Design review of the part built by this model. Coordinates are the model's own, in mm. A direction names the side the tool comes from. Coordinates: 2 decimals unless noted, no trailing zeros. Loops run counter-clockwise (first coordinate to the right, second up) from the corner with the lowest first, then second, coordinate; pieces in that order, holes last. Notation, with made-up numbers: (76, 82) -> (133, 82) arc R34 ccw to (133, 120) -> close; hole circle Ø11 at (65, 15.25). An arc over 180 degrees is marked (long way). Use a Markdown table: item, result. Add a question column.
Q1. For faces 1 (the face through (5, 5, 0)), 2 (the face through (5, -0.053, 7)), 3 (the face through (5, 10.947, 7)), 4 (the face through (10.885, 1.234, 7.395)), 5 (the face through (-0.8, 1.17, 7.4)), list the 3-axis set-ups (+Z, -Z, +X, -X, +Y, -Y) from which the entire face can be reached by the end or side of a thin tool; tool diameter is ignored.
Q2. Clearance check with flat-ended pins moving along their axes: pin 1 Ø8 at (y, z) = (-0.5, 8.5) entering from +X; pin 2 Ø1.5 at (x, z) = (0, 11) entering from +Y; pin 3 Ø4.5 at (x, z) = (4, 8.5) entering from +Y; pin 4 Ø6 at (y, z) = (-6, 7) entering from +X. State where each tip first meets the part, or that it passes through.
Q3. Take a section at A-A on z = 11. Write out the cut boundary in (x, y).
Q4. Draft analysis for pull direction X (two halves, no side actions). For faces 6 (the face through (5, 5, -4)), 7 (the face through (11.37, 9.06, 7.4)), 8 (the face through (9.478, 7.42, 7.395)), state which applies: pulls with the +X half, pulls with the -X half, needs draft (parallel to the pull), parting line crosses it, or undercut.
Q5. Take a section at D-D on x = 1. Write out the cut boundary in (y, z).
Q6. Take a section at B-B on x = -2.5. Write out the cut boundary in (y, z), plus the area to 3 significant figures.
Q7. Take a section at C-C on y = -3.5. Write out the cut boundary in (x, z).
Q8. For probe 1 along Y at (x, z) = (4, 5.5); probe 2 along Z at (x, y) = (4.5, -5.5); probe 3 along Y at (x, z) = (0.5, 3.25), list the stretches that pass through material, from the lowest coordinate up.
Solid Edge part; units mm, degrees
sketch "Sketch1" plane through (0, 0, 0) normal (0, 0, 1) x (1, 0, 0)
  arc A0 (-2.9781, 4.4363) -> (3.0001, 10.9473) centre (3.0001, 4.9473) cw
  line L0 (3.0001, 10.9473) -> (7.0001, 10.9473)
  arc A1 (7.0001, 10.9473) -> (12.9783, 4.4363) centre (7.0001, 4.9473) cw
  arc A2 (12.9783, 4.4363) -> (10.4883, 0.9473) centre (7.1717, 5.9473) cw
  arc A3 (10.4883, 0.9473) -> (7.1717, -0.0527) centre (7.1717, 5.9473) cw
  line L1 (7.1717, -0.0527) -> (2.8286, -0.0527)
  arc A4 (2.8286, -0.0527) -> (-0.4881, 0.9473) centre (2.8286, 5.9473) cw
  arc A5 (-0.4881, 0.9473) -> (-2.9781, 4.4363) centre (2.8286, 5.9473) cw
  line L2 (3.0001, 8.4473) -> (7.0001, 8.4473)
  arc A6 (7.0001, 8.4473) -> (10.4991, 4.8617) centre (7.0001, 4.9473) cw
  arc A7 (10.4991, 4.8617) -> (9.1064, 3.0306) centre (7.1717, 5.9473) cw
  arc A8 (9.1064, 3.0306) -> (7.1717, 2.4473) centre (7.1717, 5.9473) cw
  line L3 (7.1717, 2.4473) -> (2.8286, 2.4473)
  arc A9 (2.8286, 2.4473) -> (0.8939, 3.0306) centre (2.8286, 5.9473) cw
  arc A10 (0.8939, 3.0306) -> (-0.4988, 4.8617) centre (2.8286, 5.9473) cw
  arc A11 (-0.4988, 4.8617) -> (3.0001, 8.4473) centre (3.0001, 4.9473) cw
extrude "Protrusion1" add sketch "Sketch1" along normal blind 15
sketch "Sketch2" plane through (5.0001, 5.4473, 0) normal (0, 0, -1) x (1, 0, 0)
  circle A0 centre (-0.0852, 0.1989) radius 15.3143
extrude "ExtrudedProtrusion_2" add sketch "Sketch2" along normal blind 4
Answer list:
| question | item | result |
|---|---|---|
| 1 | face 1 | +Z |
| 1 | face 2 | +Z, +X, -X, -Y |
| 1 | face 3 | +Z, +X, -X, +Y |
| 1 | face 4 | +Z, +X, -Y |
| 1 | face 5 | +Z, -X, -Y |
| 2 | pin 1 | x = 12.65 |
| 2 | pin 2 | y = 10.51 |
| 2 | pin 3 | y = 10.95 |
| 2 | pin 4 | through |
| 3 | outline | (-2.98, 4.44) arc R6 ccw to (2.83, -0.05) -> (7.17, -0.05) arc R6 ccw to (12.98, 4.44) arc R6 ccw to (7, 10.95) -> (3, 10.95) arc R6 ccw to start; hole (-0.5, 4.86) arc R3.5 ccw to (2.83, 2.45) -> (7.17, 2.45) arc R3.5 ccw to (10.5, 4.86) arc R3.5 ccw to (7, 8.45) -> (3, 8.45) arc R3.5 ccw to start |
| 4 | face 6 | needs draft |
| 4 | face 7 | pulls with the +X half |
| 4 | face 8 | undercut |
| 5 | outline | (-9.56, -4) -> (20.05, -4) -> (20.05, 0) -> (10.6, 0) -> (10.6, 15) -> (7.82, 15) -> (7.82, 0) -> (2.96, 0) -> (2.96, 15) -> (0.23, 15) -> (0.23, 0) -> (-9.56, 0) -> close |
| 6 | outline | (-8.15, -4) -> (18.65, -4) -> (18.65, 0) -> (7.34, 0) -> (7.34, 15) -> (3.19, 15) -> (3.19, 0) -> (-8.15, 0) -> close |
| 6 | area | 170 mm² |
| 7 | outline | (-7.65, -4) -> (17.48, -4) -> (17.48, 0) -> (-7.65, 0) -> close |
| 8 | probe 1 | -0.05 to 2.45, 8.45 to 10.95 |
| 8 | probe 2 | -4 to 0 |
| 8 | probe 3 | 0.42 to 3.33, 7.4 to 10.4 |
